Build history of the part. All positions in model axes, mm. Face numbers are marked on the shaded views. Coordinates: 2 decimals unless noted, no trailing zeros. Write each loop counter-clockwise with the first axis right and the second up, starting at its lowest first coordinate (ties: lowest second). Pieces come first, ordered by that corner, then holes.
from build123d import *

# Parameters (mm, degrees)
SKICA1_R                     = 52.5
SKICA1_R_2                   = 51
P_IDAT_VYSUNUT_M1_DEPTH      = 26
P_IDAT_VYSUNUT_M1_DEPTH_BACK = 3
SKICA1_3_R                   = 51
P_IDAT_VYSUNUT_M3_DEPTH      = 3
ODEBRAT_START                = 2.5
ODEBRAT_VYSUNUT_M1_DEPTH     = 6
ODEBRAT_START_2              = 9.5
ODEBRAT_VYSUNUT_M2_DEPTH     = 11
ZAOBLIT1_R                   = 0.5
ZAOBLIT2_R                   = 0.5
ODEBRAT_START_3              = 11
ODEBRAT_VYSUNUT_M3_DEPTH     = 10
ZAOBLIT3_R                   = 0.5
SKICA6_W                     = 5.5
SKICA6_H                     = 2.5
ODEBRAT_VYSUNUT_M4_DEPTH     = 5


with BuildPart() as part:
    # Skica1 → P_idat vysunut_m1 (new body, two sides)
    with BuildSketch(Plane(origin=(0, 0, 0), x_dir=(1, 0, 0), z_dir=(0, 1, 0))) as p_idat_vysunut_m1_sk:
        Circle(SKICA1_R)
        Circle(SKICA1_R_2, mode=Mode.SUBTRACT)
    extrude(amount=P_IDAT_VYSUNUT_M1_DEPTH)
    extrude(p_idat_vysunut_m1_sk.sketch, amount=-P_IDAT_VYSUNUT_M1_DEPTH_BACK)

    # Skica1_3 → P_idat vysunut_m3 (add)
    with BuildSketch(Plane(origin=(0, 0, 0), x_dir=(1, 0, 0), z_dir=(0, 1, 0))):
        Circle(SKICA1_3_R)
    extrude(amount=-P_IDAT_VYSUNUT_M3_DEPTH)

    # Skica3 → Odebrat vysunut_m1 (cut)
    with BuildSketch(Plane(origin=(0, 0, 0), x_dir=(1, 0, 0), z_dir=(0, 1, 0)).offset(ODEBRAT_START)):
        Polygon((-24.5, -44.729744019), (-25.943243016, -46.771079267), (-35.443243016, -40.054490866), (-34, -38.013155617), align=None)
    extrude(amount=ODEBRAT_VYSUNUT_M1_DEPTH, mode=Mode.SUBTRACT)

    # Skica4 → Odebrat vysunut_m2 (cut)
    with BuildSketch(Plane(origin=(0, 0, 0), x_dir=(1, 0, 0), z_dir=(0, 1, 0)).offset(ODEBRAT_START_2)):
        Polygon((-16.5, -48.257123826), (-17.470460132, -50.561078499), (-23.970460132, -47.823181379), (-23, -45.519226707), align=None)
    extrude(amount=ODEBRAT_VYSUNUT_M2_DEPTH, mode=Mode.SUBTRACT)

    # Zaoblit1
    zaoblit1_edges = [part.edges().sort_by_distance(p)[0] for p in [
        (-34.435735274, 8.5, 38.629463311),
        (-24.935735274, 2.5, 45.346051713),
        (-24.935735274, 8.5, 45.346051713),
        (-34.435735274, 2.5, 38.629463311),
    ]]
    fillet(zaoblit1_edges, radius=ZAOBLIT1_R)

    # Zaoblit2
    zaoblit2_edges = [part.edges().sort_by_distance(p)[0] for p in [
        (-16.791816548, 20.5, 48.949921063),
        (-23.291816548, 20.5, 46.212023944),
        (-23.291816548, 9.5, 46.212023944),
        (-16.791816548, 9.5, 48.949921063),
    ]]
    fillet(zaoblit2_edges, radius=ZAOBLIT2_R)

    # Skica5 → Odebrat vysunut_m3 (cut)
    with BuildSketch(Plane(origin=(0, 0, 0), x_dir=(1, 0, 0), z_dir=(0, 1, 0)).offset(ODEBRAT_START_3)):
        Polygon((2.5, 50.938688636), (2.734091597, 53.438688636), (7.234091597, 53.017323761), (7, 50.517323761), align=None)
    extrude(amount=ODEBRAT_VYSUNUT_M3_DEPTH, mode=Mode.SUBTRACT)

    # Zaoblit3
    zaoblit3_edges = [part.edges().sort_by_distance(p)[0] for p in [
        (2.569988396, 21, -51.686135324),
        (7.069988396, 21, -51.264770449),
        (7.069988396, 11, -51.264770449),
        (2.569988396, 11, -51.686135324),
    ]]
    fillet(zaoblit3_edges, radius=ZAOBLIT3_R)

    # Skica6 → Odebrat rotac_1 (revolve, cut)
    with BuildSketch(Plane(origin=(0, 16, 0), x_dir=(1, 0, 0), z_dir=(0, 1, 0))):
        with Locations((-2.75, -51.25)):
            Rectangle(SKICA6_W, SKICA6_H)
    revolve(axis=Axis((0, 16, -58.211377778), (0, 0, 1)), mode=Mode.SUBTRACT)

    # Skica7 → Odebrat vysunut_m4 (cut)
    with BuildSketch(Plane(origin=(0, 16, 0), x_dir=(1, 0, 0), z_dir=(0, 1, 0))):
        Polygon((46.914816423, 20), (44.730924047, 24.497845494), (46.979846795, 25.589791682), (49.16373917, 21.091946188), align=None)
    extrude(amount=-ODEBRAT_VYSUNUT_M4_DEPTH, mode=Mode.SUBTRACT)


solid = part.part
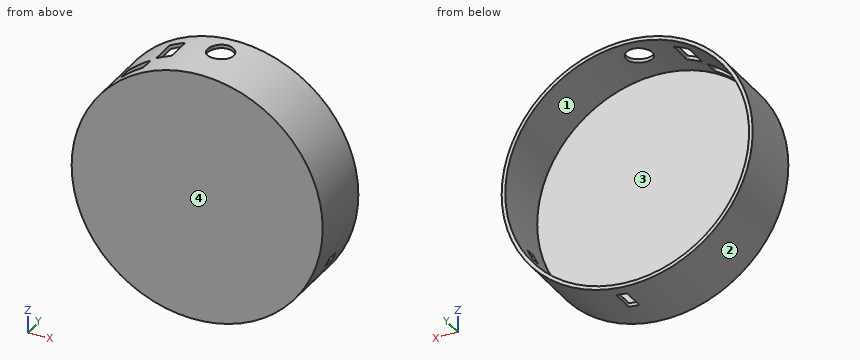
(1) Flat gauge pins, fed straight in: P1, Ø2, axis at y = 17, z = -31.5, coming from the +X side; P2, Ø3, axis at x = 37, y = 20, coming from the +Z side; P3, Ø8, axis at x = 8, y = 15, coming from the +Z side. Where does each tip first touch, or does it go through?
(2) Slice it at A-A, the plane x = 0. List the corners of the cut face in (y, z), and give its area (4 significant figures).
(3) Slice it at B-B, the plane y = 13.5. List the corners of the cut face in (x, z), and give its area (3 significant figures).
(4) Two-plate mould, pull along Z, no slides. Class the marked faces 1, 2, 3 and 4: pulls with the +Z half, pulls with the -Z half, needs draft (parallel to the pull), parting line crosses it, or undercut.
(5) Slice it at C-C, the plane z = 0. List the corners of the cut face in (x, y).
(6) Probe L1, parallel to X at y = 15.25, z = 0; L2, parallel to Y at x = 0, z = 51.65; L3, parallel to Y at x = -5, z = 30. List the from-to ranges inside material, lowest first.
(7) Slice it at D-D, the plane x = 43. List the corners of the cut face in (y, z).
Results:
1. P1: stops at x = 42.73
1. P2: stops at z = 38.68
1. P3: stops at z = 52.3
2. outline: (-3, -52.5) - (26, -52.5) - (26, -51) - (0, -51) - (0, 51) - (10.5, 51) - (10.5, 52.5) - (-3, 52.5) - close; (21.5, 51) - (26, 51) - (26, 52.5) - (21.5, 52.5) - close
2. area: 376.5 mm2
3. outline: (-23.58, 46.9) arc R52.5 ccw to (2.64, -52.43) - (2.5, -50.94) arc R51 cw to (-23, 45.52) - close; (-17.08, 49.64) - (-16.5, 48.26) arc R51 cw to (-4.9, 50.76) - (-4.9, 52.27) arc R52.5 ccw to start; (4.9, 50.76) arc R51 cw to (46.91, -20) - (48.27, -20.66) arc R52.5 ccw to (4.9, 52.27) - close; (7, -50.52) - (7.14, -52.01) arc R52.5 ccw to (46.08, -25.15) - (44.73, -24.5) arc R51 cw to start
3. area: 448 mm2
4. face 1: undercut
4. face 2: parting line crosses it
4. face 3: undercut
4. face 4: needs draft
5. outline: (-52.5, -3) - (52.5, -3) - (52.5, 26) - (51, 26) - (51, 0) - (-51, 0) - (-51, 26) - (-52.5, 26) - close
6. L1: x = -52.5 to -51, 51 to 52.5
6. L2: y = -3 to 10.5, 21.5 to 26
6. L3: y = -3 to 0
7. outline: (-3, -30.12) - (26, -30.12) - (26, -27.42) - (0, -27.42) - (0, 27.42) - (26, 27.42) - (26, 30.12) - (-3, 30.12) - close
